Could you check a few things on this model? Use its own coordinates, in mm. Face numbers are marked on the shaded views. A direction names the side the tool comes from. Round coordinates to 2 decimals unless told otherwise and drop trailing zeros. Loops run counter-clockwise (first coordinate to the right, second up) from the corner with the lowest first, then second, coordinate; pieces in that order, holes last. Notation, with made-up numbers: (2, -19.75) -> (47, -19.75) arc R29 cw to (47, 12.25) -> close; hole circle Ø3 at (44.5, 36). An arc over 180 degrees is marked (long way). One line per item, written item: value.
```python
from build123d import *

# Parameters (mm, degrees)
SKETCH1_R            = 3.25
BOSS_EXTRUDE1_DEPTH  = 8.5
SKETCH3_W            = 65
SKETCH3_H            = 51.25
BOSS_EXTRUDE2_DEPTH  = 2.5
SKETCH4_W            = 7.6
SKETCH4_H            = 30.6
BOSS_EXTRUDE3_DEPTH  = 14
SKETCH5_R            = 3.25
BOSS_EXTRUDE4_DEPTH  = 8.5
SKETCH6_W            = 25.75
SKETCH6_H            = 2.5
BOSS_EXTRUDE5_DEPTH  = 12.25
SKETCH8_R            = 3.25
BOSS_EXTRUDE9_DEPTH  = 8.5
SKETCH9_W            = 20.5
SKETCH9_H            = 2.5
BOSS_EXTRUDE10_DEPTH = 12.25
SKETCH10_W           = 20.5
SKETCH10_H           = 12.25
CUT_EXTRUDE1_DEPTH   = 0.1
SKETCH12_W           = 25.75
SKETCH12_H           = 12.25
BOSS_EXTRUDE11_DEPTH = 0.1
SKETCH14_W           = 14
SKETCH14_H           = 30.6
BOSS_EXTRUDE12_DEPTH = 0.1
SKETCH15_R           = 1.5
CUT_EXTRUDE2_DEPTH   = 3.5
SKETCH16_R           = 1.75
CUT_EXTRUDE3_DEPTH   = 3.5
SKETCH17_W           = 16
SKETCH17_H           = 16
BOSS_EXTRUDE13_DEPTH = 1.25
SKETCH18_W           = 16
SKETCH18_H           = 17.25
BOSS_EXTRUDE14_DEPTH = 1.25


with BuildPart() as part:
    # Sketch1 → Boss-Extrude1 (new body)
    with BuildSketch(Plane.XY):
        with Locations((-17.5, -3)):
            Circle(SKETCH1_R)
    extrude(amount=BOSS_EXTRUDE1_DEPTH)

    # Sketch3 → Boss-Extrude2 (add)
    with BuildSketch(Plane.XY):
        Rectangle(SKETCH3_W, SKETCH3_H)
    extrude(amount=-BOSS_EXTRUDE2_DEPTH)

    # Sketch4 → Boss-Extrude3 (add)
    with BuildSketch(Plane.XY):
        with Locations((28.7, 0)):
            Rectangle(SKETCH4_W, SKETCH4_H)
    extrude(amount=BOSS_EXTRUDE3_DEPTH)

    # Sketch5 → Boss-Extrude4 (add)
    with BuildSketch(Plane.XY):
        with Locations((-10.25, 4)):
            Circle(SKETCH5_R)
    extrude(amount=BOSS_EXTRUDE4_DEPTH)

    # Sketch6 → Boss-Extrude5 (add)
    with BuildSketch(Plane.XY):
        with Locations((-1.875, 24.375)):
            Rectangle(SKETCH6_W, SKETCH6_H)
    extrude(amount=BOSS_EXTRUDE5_DEPTH)

    # Sketch8 → Boss-Extrude9 (add)
    with BuildSketch(Plane.XY):
        with Locations((-9.5, 19.87)):
            Circle(SKETCH8_R)
    extrude(amount=BOSS_EXTRUDE9_DEPTH)

    # Sketch9 → Boss-Extrude10 (add)
    with BuildSketch(Plane.XY):
        with Locations((4.25, -24.375)):
            Rectangle(SKETCH9_W, SKETCH9_H)
    extrude(amount=BOSS_EXTRUDE10_DEPTH)

    # Sketch10 → Cut-Extrude1 (cut)
    with BuildSketch(Plane.XZ.offset(25.625)):
        with Locations((4.25, 6.125)):
            Rectangle(SKETCH10_W, SKETCH10_H)
    extrude(amount=-CUT_EXTRUDE1_DEPTH, mode=Mode.SUBTRACT)

    # Sketch12 → Boss-Extrude11 (add)
    with BuildSketch(Plane(origin=(0, 25.625, 0), x_dir=(1, 0, 0), z_dir=(0, 1, 0))):
        with Locations((-1.875, -6.125)):
            Rectangle(SKETCH12_W, SKETCH12_H)
    extrude(amount=BOSS_EXTRUDE11_DEPTH)

    # Sketch14 → Boss-Extrude12 (add)
    with BuildSketch(Plane(origin=(32.5, 0, 0), x_dir=(0, 0, -1), z_dir=(1, 0, 0))):
        with Locations((-7, 0)):
            Rectangle(SKETCH14_W, SKETCH14_H)
    extrude(amount=BOSS_EXTRUDE12_DEPTH)

    # Sketch15 → Cut-Extrude2 (cut, through all)
    with BuildSketch(Plane.XY):
        with Locations((-29, 22.125)):
            Circle(SKETCH15_R)
    extrude(amount=-CUT_EXTRUDE2_DEPTH, mode=Mode.SUBTRACT)

    # Sketch16 → Cut-Extrude3 (cut, through all)
    with BuildSketch(Plane.XY):
        with Locations((-21.25, -22.125)):
            Circle(SKETCH16_R)
    extrude(amount=-CUT_EXTRUDE3_DEPTH, mode=Mode.SUBTRACT)

    # Sketch17 → Boss-Extrude13 (add)
    with BuildSketch(Plane.XY):
        with Locations((7.5, 14.875)):
            Rectangle(SKETCH17_W, SKETCH17_H)
    extrude(amount=BOSS_EXTRUDE13_DEPTH)

    # Sketch18 → Boss-Extrude14 (add)
    with BuildSketch(Plane.XY):
        with Locations((7.5, -11.375)):
            Rectangle(SKETCH18_W, SKETCH18_H)
    extrude(amount=BOSS_EXTRUDE14_DEPTH)


solid = part.part
```
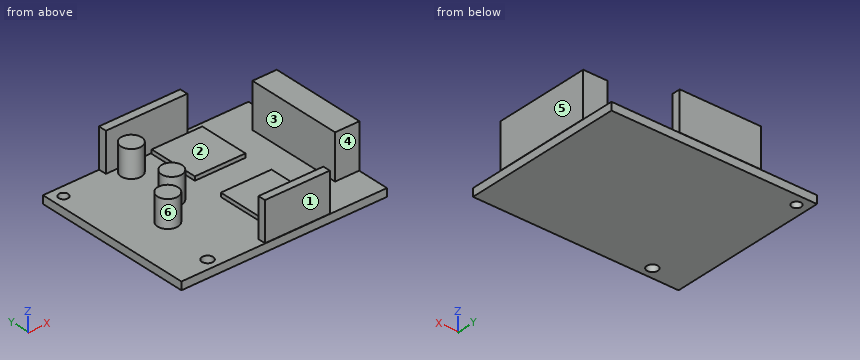
Item 1: Will these pins go through, and if not, where does the flat tip stop? pin 1 Ø8 at (x, y) = (-18.5, 18) entering from +Z; pin 2 Ø7 at (x, y) = (-18, -3) entering from +Z; pin 3 Ø0.7 at (x, y) = (4.5, -24.5) entering from +Z.
Output:
pin 1: stops at z = 0
pin 2: stops at z = 8.5
pin 3: stops at z = 12.25
Item 2: For the marked faces 1, 2 and 3, which set-ups out of +Z, -Z, +X, -X, +Y, -Y let a thin tool reach every point of the face, with its end or its side?
Output:
face 1: +Z, +X, -X, -Y
face 2: +Z
face 3: +Z, +Y, -Y
Item 3: If we section it at D-D on y = 19.87: List the corners of the cut face in (x, z) for me, plus the area to 3 significant figures.
Output:
outline: (-32.5, -2.5) -> (32.5, -2.5) -> (32.5, 0) -> (15.5, 0) -> (15.5, 1.25) -> (-0.5, 1.25) -> (-0.5, 0) -> (-6.25, 0) -> (-6.25, 8.5) -> (-12.75, 8.5) -> (-12.75, 0) -> (-32.5, 0) -> close
area: 238 mm²
Item 4: I need wall thicknesses on line 1 (Y direction, x = -29, z = -1.9) (3 decimals); line 2 (Y direction, x = -21.25, z = -0.6) (3 decimals); line 3 (Y direction, x = 3.5, z = -1.5) (3 decimals). Which ranges of each line are inside material? Lowest first, please. Write a range as from..to.
Output:
line 1: y = -25.625..20.625, 23.625..25.625
line 2: y = -25.625..-23.875, -20.375..25.625
line 3: y = -25.625..25.625
Item 5: If we mould it in two halves opening along X, with no side actions, what happens to the marked faces 4, 5 and 6? For each: released by +X, released by -X, zero draft, split by the parting line, or undercut.
Output:
face 4: zero draft
face 5: released by +X
face 6: undercut
Item 6: If we section it at A-A on z = 11: List the corners of the cut face in (x, y) for me (3 decimals).
Output:
outline: (-14.75, 23.125) -> (11, 23.125) -> (11, 25.725) -> (-14.75, 25.725) -> close; (-6, -25.525) -> (14.5, -25.525) -> (14.5, -23.125) -> (-6, -23.125) -> close; (24.9, -15.3) -> (32.6, -15.3) -> (32.6, 15.3) -> (24.9, 15.3) -> close
Item 7: If we section it at C-C on z = 3.5: List the corners of the cut face in (x, y) for me (3 decimals).
Output:
outline: circle Ø6.5 at (-17.5, -3); (-14.75, 23.125) -> (11, 23.125) -> (11, 25.725) -> (-14.75, 25.725) -> close; circle Ø6.5 at (-10.25, 4); circle Ø6.5 at (-9.5, 19.87); (-6, -25.525) -> (14.5, -25.525) -> (14.5, -23.125) -> (-6, -23.125) -> close; (24.9, -15.3) -> (32.6, -15.3) -> (32.6, 15.3) -> (24.9, 15.3) -> close
Item 8: If we section it at B-B on x = -17.5: List the corners of the cut face in (y, z) for me (3 decimals).
Output:
outline: (-25.625, -2.5) -> (25.625, -2.5) -> (25.625, 0) -> (0.25, 0) -> (0.25, 8.5) -> (-6.25, 8.5) -> (-6.25, 0) -> (-25.625, 0) -> close
